from build123d import *

# Parameters (mm, degrees)
F0_W      = 50
F0_H      = 20
F1_DEPTH  = 10
F2_W      = 50
F2_H      = 30
F3_DEPTH  = 10
F4_R      = 3.8263869055
F5_DEPTH  = 28.956
F10_W     = 5.2931006998
F10_H     = 2.3875854537
F10_W_2   = 5.2931062877
F11_DEPTH = 20.001
F12_R     = 1.7676057038
F12_R_2   = 2.0091255021
F13_DEPTH = 3.81
F14_R     = 5.9356630849
F14_R_2   = 5.9251919842
F15_DEPTH = 1.778
F16_R     = 2.9121930079
F16_R_2   = 2.9560346156
F17_DEPTH = 2.032


# Not quite as in the source:
# - a pattern or mirror of a feature is missing from the dataset's text; its kind, count and spacing are read off the source's solid


with BuildPart() as f1:
    # F0 (on Front) → F1 (new body, symmetric)
    with BuildSketch(Plane.XZ):
        Rectangle(F0_W, F0_H)
    extrude(amount=F1_DEPTH, both=True)

    # F2 (on Top) → F3 (join)
    with BuildSketch(Plane.XY):
        Rectangle(F2_W, F2_H)
    extrude(amount=F3_DEPTH)

    # F4 (on Right) → F5 (join, symmetric)
    with BuildSketch(Plane.YZ):
        with Locations((0, -5.3208619356)):
            Circle(F4_R)
    extrude(amount=F5_DEPTH, both=True)

    # F6 (on face) → F7 (revolve)
    with BuildSketch(Plane(origin=(-28.956, 0, 0), x_dir=(0, -1, 0), z_dir=(-1, 0, 0))):
        with BuildLine():
            Line((0, -1.5713692232), (0, -9.0703546481))
            ThreePointArc((0, -9.0703546481), (3.7494927125, -5.3208619356), (0, -1.5713692232))
        make_face()
    revolve(axis=Axis((-28.956, 0, -5.2824148391), (0, 0, -1)))

    # F8 (on face) → F9 (revolve)
    with BuildSketch(Plane.YZ.offset(28.956)):
        with BuildLine():
            Line((0, -1.6739376972), (0, -8.967786174))
            ThreePointArc((0, -8.967786174), (3.6469242384, -5.3208619356), (0, -1.6739376972))
        make_face()
    revolve(axis=Axis((28.956, 0, -5.3208619356), (0, 0, -1)))

    # F10 (on face) → F11 (cut, through all)
    with BuildSketch(Plane.XY.offset(10)):
        with Locations((-22.3534496501, 13.8062072732)):
            Rectangle(F10_W, F10_H)
        with Locations((22.3534468561, 13.8062072732)):
            Rectangle(F10_W_2, F10_H)
    extrude(amount=-F11_DEPTH, mode=Mode.SUBTRACT)

    # F12 (on face) → F13 (join)
    with BuildSketch(Plane.XZ.offset(10)):
        with Locations((-18.9186222851, -10)):
            Circle(F12_R)
        with Locations((16.5537931025, -10)):
            Circle(F12_R_2)
    f13 = extrude(amount=F13_DEPTH)

    # F13_copies: F13 across plane
    add(f13.mirror(Plane.ZX))

    # F14 (on face) → F15 (join)
    with BuildSketch(Plane.XZ.offset(13.81)):
        with Locations((-18.9186222851, -10)):
            Circle(F14_R)
        with Locations((16.3567233831, -10.247586295)):
            Circle(F14_R_2)
    f15 = extrude(amount=F15_DEPTH)

    # F15_copies: F15 across plane
    add(f15.mirror(Plane.ZX))

    # F16 (on face) → F17 (join)
    with BuildSketch(Plane.XZ.offset(15.588)):
        with Locations((-18.9186222851, -10)):
            Circle(F16_R)
        with Locations((16.1596573889, -10.247586295)):
            Circle(F16_R_2)
    f17 = extrude(amount=F17_DEPTH)

    # F17_copies: F17 across plane
    add(f17.mirror(Plane.ZX))


solid = f1.part
Source: CAD feature listing. Evaluate the final solid. Frame: model axes, mm. A direction names the side the tool comes from. Coordinates: 2 decimals unless noted, no trailing zeros. Loops run counter-clockwise (first coordinate to the right, second up) from the corner with the lowest first, then second, coordinate; pieces in that order, holes last. Notation, with made-up numbers: (13.5, 21) - (61.5, 21) arc R16 ccw to (61.5, 28) - close; hole circle Ø11 at (31.25, -18). An arc over 180 degrees is marked (long way). Return JSON: item names as keys, results as strings.
Q1. Access query for faces 1 (the flat face through (0, 15, 5)), 2 (the cylindrical face through (-20.3, 11.9, -11.1)), 3 (the flat face through (19, 15.588, -13)), 4 (the flat face through (0, 13, 0)), 5 (the cylindrical face through (22.01, -14.69, -8.47)). Directions: +Z, -Z, +X, -X, +Y, -Y. A direction counts if a zero-diameter tool reaches every point of the face in a straight line with its end or side. Return the directions, or none.
Results:
{"face 1": "+Z, +X, -X, +Y", "face 2": "none", "face 3": "+Y", "face 4": "+X, -X, +Y", "face 5": "-Y"}
Q2. Mould query, pull axis X, two halves, no side actions, for faces 6 (the cylindrical face through (-23.63, 14.69, -13.61)), 7 (the flat face through (25, -1, 2)), 8 (the flat face through (-25, -1, 2)). Classes: released by +X, released by -X, zero draft, split by the parting line, or undercut.
Results:
{"face 6": "undercut", "face 7": "released by +X", "face 8": "released by -X"}
Q3. Material intervals for line 1 along Y through (x, z) = (-16, -8); line 2 along Z through (x, y) = (1, -11); line 3 along Z through (x, y) = (-6.5, -3.5), sorted ascending.
Results:
{"line 1": "-15.59 to -13.81, -10 to 10, 13.81 to 15.59", "line 2": "0 to 10", "line 3": "-10 to 10"}
Q4. Contact query for flat-ended pins moving along their axis: P1, Ø2.5, axis at x = -2, y = -13.5, coming from the -Z side; P2, Ø2.5, axis at x = 21.5, z = 4.5, coming from the +Y side; P3, Ø4, axis at x = 3, z = -3.5, coming from the -Y side. Output: stop coordinate, or through.
Results:
{"P1": "z = 0", "P2": "y = 12.61", "P3": "y = -10"}
Q5. Section B-B, the plane x = -2. Return loops of the section in (y, z).
Results:
{"outline": "(-15, 0) - (-10, 0) - (-10, -10) - (10, -10) - (10, 0) - (15, 0) - (15, 10) - (-15, 10) - close"}
Q6. Section D-D, the plane z = -14. Return loops of the section in (x, y), plus the area to 3 significant figures.
Results:
{"outline": "(-23.3, -15.59) - (-14.53, -15.59) - (-14.53, -13.81) - (-23.3, -13.81) - close; (-23.3, 13.81) - (-14.53, 13.81) - (-14.53, 15.59) - (-23.3, 15.59) - close; (11.77, -15.59) - (20.94, -15.59) - (20.94, -13.81) - (11.77, -13.81) - close; (11.77, 13.81) - (20.94, 13.81) - (20.94, 15.59) - (11.77, 15.59) - close", "area": "63.8 mm2"}
Q7. Section C-C, the plane y = 0. Return loops of the section in (x, z), plus the area to 3 significant figures.
Results:
{"outline": "(-28.96, -9.15) - (-25, -9.15) - (-25, -10) - (25, -10) - (25, -9.15) - (28.96, -9.15) - (28.96, -8.97) arc R3.65 ccw to (28.96, -1.67) - (28.96, -1.49) - (25, -1.49) - (25, 10) - (-25, 10) - (-25, -1.49) - (-28.96, -1.49) - (-28.96, -1.57) arc R3.75 ccw to (-28.96, -9.07) - close", "area": "1,100 mm2"}
Q8. Section A-A, the plane z = -6.25. Give the number of separate pieces and of enclosed holes in the cut face, plus the area to 3 significant figures.
Results:
{"separate pieces": "5", "enclosed holes": "0", "area": "1,160 mm2"}
